Read the model definition and answer for the solid it produces. Units are mm, in the model's axes. A direction names the side the tool comes from. Coordinates: 2 decimals unless noted, no trailing zeros. Order: outer loops, then holes, each group sorted by start corner. A loop starts at its lowest first (then second) coordinate and runs counter-clockwise, first axis right, second up. Notation, with made-up numbers: (8, 82.5) -> (53, 82.5) arc R19 cw to (53, 109.5) -> close; hole circle Ø2 at (-27.75, 31.5). An arc over 180 degrees is marked (long way). Answer in a Markdown table with one row per item.
from build123d import *

# Parameters (mm, degrees)
CSK_FOR_M2_5_COUNTERSUNK_FLAT_HEAD_S_2_COUNT = 2
CSK_FOR_M2_5_COUNTERSUNK_FLAT_HEAD_S_2_PITCH = 21.920310217
CSK_FOR_M2_5_COUNTERSUNK_FLAT_HEAD_S_3_COUNT = 2
CSK_FOR_M2_5_COUNTERSUNK_FLAT_HEAD_S_3_PITCH = 31
CSK_FOR_M2_5_COUNTERSUNK_FLAT_HEAD_S_4_COUNT = 2
CSK_FOR_M2_5_COUNTERSUNK_FLAT_HEAD_S_4_PITCH = 21.920310217


with BuildPart() as part:
    # Sketch1 → Revolve1 (revolve)
    with BuildSketch(Plane.XY):
        Polygon((-24.5, 0), (-12.5, 0), (-12.5, 1), (-18.8, 1), (-18.8, 2), (-24.5, 2), (-24.5, 1.005), (-24, 1.005), (-24, 0.995), (-24.5, 0.995), align=None)
    revolve(axis=Axis((0, 0, 0), (0, 1, 0)))

    # Sketch2 → CSK for M2.5 Countersunk Flat Head Screw1 (revolve, cut)
    with BuildSketch(Plane(origin=(0, 1, -15.5), x_dir=(0, 0, 1), z_dir=(1, 0, 0))):
        Polygon((0, 0), (0, 1), (1.55, 1), (1.55, 0.75), (2.3, 0), align=None)
    csk_for_m2_5_countersunk_flat_head_screw = revolve(axis=Axis((0, 7.35, -15.5), (0, -1, 0)), mode=Mode.SUBTRACT)

    # CSK for M2.5 Countersunk Flat Head S 2: CSK for M2.5 Countersunk Flat Head Screw1 ×2
    with Locations(*[Vector(-0.707106781, 0, 0.707106781) * (i * CSK_FOR_M2_5_COUNTERSUNK_FLAT_HEAD_S_2_PITCH) for i in range(1, CSK_FOR_M2_5_COUNTERSUNK_FLAT_HEAD_S_2_COUNT)]):
        add(csk_for_m2_5_countersunk_flat_head_screw, mode=Mode.SUBTRACT)

    # CSK for M2.5 Countersunk Flat Head S 3: CSK for M2.5 Countersunk Flat Head Screw1 ×2
    with Locations(*[(0, 0, i * CSK_FOR_M2_5_COUNTERSUNK_FLAT_HEAD_S_3_PITCH) for i in range(1, CSK_FOR_M2_5_COUNTERSUNK_FLAT_HEAD_S_3_COUNT)]):
        add(csk_for_m2_5_countersunk_flat_head_screw, mode=Mode.SUBTRACT)

    # CSK for M2.5 Countersunk Flat Head S 4: CSK for M2.5 Countersunk Flat Head Screw1 ×2
    with Locations(*[Vector(0.707106781, 0, 0.707106781) * (i * CSK_FOR_M2_5_COUNTERSUNK_FLAT_HEAD_S_4_PITCH) for i in range(1, CSK_FOR_M2_5_COUNTERSUNK_FLAT_HEAD_S_4_COUNT)]):
        add(csk_for_m2_5_countersunk_flat_head_screw, mode=Mode.SUBTRACT)


solid = part.part
Q1. Consider line 1 (Z direction, x = 0, y = 0.8); line 2 (Z direction, x = -0.5, y = 0.35); line 3 (X direction, y = 0.5, z = -1). Determine where each line is inside the solid, lowest interval first.
Outcome:
| item | result |
|---|---|
| line 1 | -24.5 to -17.6, -13.4 to -12.5, 12.5 to 13.4, 17.6 to 24.5 |
| line 2 | -24.49 to -17.07, -13.93 to -12.49, 12.49 to 13.93, 17.07 to 24.49 |
| line 3 | -24.48 to -17, -14 to -12.46, 12.46 to 14, 17 to 24.48 |
Q2. For faces 4 (the face through (-11.923, 0.507, 3.755)), 5 (the face through (4.08, 1.51, -18.35)), determine the directions among +Z, -Z, +X, -X, +Y, -Y from which every point of the face is accessible in a straight line to the end or side of a thin tool.
Outcome:
| item | result |
|---|---|
| face 4 | +Y, -Y |
| face 5 | +Y |
Q3. The part is cut by section C-C (x = -15.5). Write down the section's boundary in (y, z) (3 decimals), then the cut area to 3 significant figures.
Outcome:
| item | result |
|---|---|
| outline | (0, -18.974) -> (0.995, -18.974) -> (0.995, -18.323) -> (1.005, -18.323) -> (1.005, -18.974) -> (2, -18.974) -> (2, -10.639) -> (1, -10.639) -> (1, -2.3) -> (0.25, -1.55) -> (0, -1.55) -> close; (0, 1.55) -> (0.25, 1.55) -> (1, 2.3) -> (1, 10.639) -> (2, 10.639) -> (2, 18.974) -> (1.005, 18.974) -> (1.005, 18.323) -> (0.995, 18.323) -> (0.995, 18.974) -> (0, 18.974) -> close |
| area | 50.9 mm² |
Q4. For a pull along Z with two mould halves and no side action, classify faces 1 (the face through (3.9, 1, -12.3)), 2 (the face through (-13.17, 0.49, 20.66)), 3 (the face through (-11, 0, -11)) as pulls with the +Z half, pulls with the -Z half, needs draft (parallel to the pull), parting line crosses it, or undercut.
Outcome:
| item | result |
|---|---|
| face 1 | undercut |
| face 2 | parting line crosses it |
| face 3 | needs draft |
Q5. The part is cut by section B-B (z = 9). Write down the section's boundary in (x, y) (3 decimals), then the cut area to 3 significant figures.
Outcome:
| item | result |
|---|---|
| outline | (-22.787, 0) -> (-8.675, 0) -> (-8.675, 1) -> (-16.506, 1) -> (-16.506, 2) -> (-22.787, 2) -> (-22.787, 1.005) -> (-22.249, 1.005) -> (-22.249, 0.995) -> (-22.787, 0.995) -> close; (8.675, 0) -> (22.787, 0) -> (22.787, 0.995) -> (22.249, 0.995) -> (22.249, 1.005) -> (22.787, 1.005) -> (22.787, 2) -> (16.506, 2) -> (16.506, 1) -> (8.675, 1) -> close |
| area | 40.8 mm² |
Q6. The part is cut by section A-A (x = 0). Give the number of separate pieces and of enclosed holes in the cut face, then the cut area to 3 significant figures.
Outcome:
| item | result |
|---|---|
| separate pieces | 4 |
| enclosed holes | 0 |
| area | 28.1 mm² |
Q7. Given pin 1 (5 mm diameter, centred on x = 9.5, z = 17, fed in from -Y); pin 2 (1.9 mm diameter, centred on x = 0, z = -15.5, fed in from -Y); pin 3 (4 mm diameter, centred on x = -15.5, z = 0, fed in from +Y); pin 4 (1 mm diameter, centred on x = -18.5, y = 0.5, fed in from -Z), each flat-ended and moving along its own axis, determine where each tip first touches the part or whether it passes through.
Outcome:
| item | result |
|---|---|
| pin 1 | y = 0 |
| pin 2 | through |
| pin 3 | y = 0.7 |
| pin 4 | z = -16.62 |
